The listing builds one solid part. Answer for the finished solid, in the listing's coordinates (mm). Coordinates: 2 decimals unless noted, no trailing zeros. Order: outer loops, then holes, each group sorted by start corner. A loop starts at its lowest first (then second) coordinate and runs counter-clockwise, first axis right, second up.
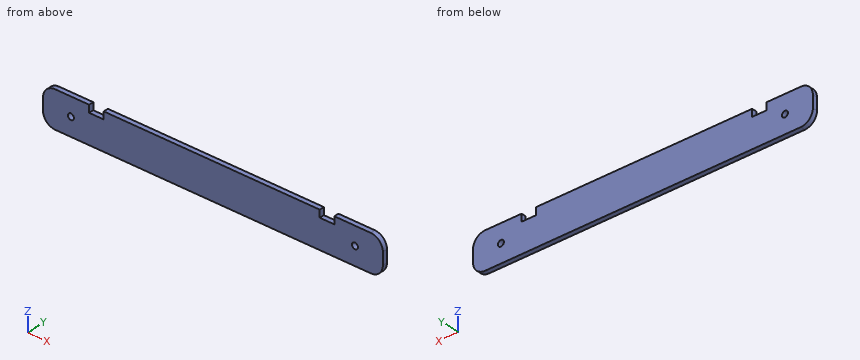
Autodesk Inventor part; units mm, degrees
ref_plane "YZ Plane" through (0, 0, 0) normal (1, 0, 0) x (0, 1, 0)
ref_plane "XZ Plane" through (0, 0, 0) normal (0, 1, 0) x (-1, 0, 0)
ref_plane "XY Plane" through (0, 0, 0) normal (0, 0, 1) x (1, 0, 0)
sketch "Sketch1" plane through (0, 0, 0) normal (0, 1, 0) x (-1, 0, 0)
  line L0 (70, 7.5) -> (-70, 7.5)
  line L1 (-70, 7.5) -> (-70, -7.5)
  line L2 (-70, -7.5) -> (70, -7.5)
  line L3 (70, -7.5) -> (70, 7.5)
  line L4 (51, 7.5) -> (51, 4.5)
  line L5 (51, 4.5) -> (45, 4.5)
  line L6 (45, 4.5) -> (45, 7.5)
  line L7 (-50, 7.5) -> (-50, 4.5)
  line L8 (-50, 4.5) -> (-44, 4.5)
  line L9 (-44, 4.5) -> (-44, 7.5)
  point P0 (0, 0)
  point P1 (58.5, 0)
  point P2 (-58.5, 0)
  point P3 (-70, 0)
  dimension "d0" = 117
  dimension "d1" = 58.5
  dimension "d2" = 140
  dimension "d3" = 70
  dimension "d4" = 7.5
  dimension "d5" = 15
  dimension "d6" = 7.5
  dimension "d7" = 6
  dimension "d8" = 3
  dimension "d9" = 7.5
  dimension "d10" = 6
  dimension "d11" = 3
  dimension "d12" = 101
extrude "Extrusion1" add sketch "Sketch1" along normal blind 2 contours L3 L2 L1 L0 L7 L8 L9 L6 L5 L4
hole "Hole1" at (-58.5, 0, 0) at (58.5, 0, 0) direction (0, 1, 0) diameter 2.5 depth 6.5
fillet "Fillet1" radius 5 4 edges at (-70, 1, 7.5) (-70, 1, -7.5) (70, 1, 7.5) (70, 1, -7.5)
properties part number "3DP_PLA_Screw_Spacing_Test_Part"
(1) Find the intervals of material crossed by probe 1 along X at (y, z) = (0.8, 0); probe 2 along X at (y, z) = (0.55, -1); probe 3 along Z at (x, y) = (58.5, 0.7), in increasing order.
(2) Find section D-D on x = -47.5. Determine the outline of the cut face in (y, z), then the cut area to 3 significant figures.
(3) Find section C-C on y = 1.3. Determine the outline of the cut face in (x, z).
(4) Find section B-B on z = 0. Determine the outline of the cut face in (x, y), then the cut area to 3 significant figures.
(5) Given pin 1 Ø0.6 at (y, z) = (1, 6) entering from -X; pin 2 Ø2 at (x, z) = (-58.5, 0) entering from -Y; pin 3 Ø3 at (x, z) = (58.5, 0) entering from -Y; pin 4 Ø0.6 at (x, y) = (46.5, 1) entering from +Z, each flat-ended and moving along its own axis, determine where each tip first touches the part or whether it passes through.
(6) Find section A-A on x = 58.5. Determine the outline of the cut face in (y, z).
Resolved:
1. probe 1: x = -70 to -59.75, -57.25 to 57.25, 59.75 to 70
1. probe 2: x = -70 to -59.25, -57.75 to 57.75, 59.25 to 70
1. probe 3: z = -7.5 to -1.25, 1.25 to 7.5
2. outline: (0, -7.5) - (2, -7.5) - (2, 4.5) - (0, 4.5) - close
2. area: 24.0 mm2
3. outline: (-70, -2.5) arc R5 ccw to (-65, -7.5) - (65, -7.5) arc R5 ccw to (70, -2.5) - (70, 2.5) arc R5 ccw to (65, 7.5) - (50, 7.5) - (50, 4.5) - (44, 4.5) - (44, 7.5) - (-45, 7.5) - (-45, 4.5) - (-51, 4.5) - (-51, 7.5) - (-65, 7.5) arc R5 ccw to (-70, 2.5) - close; hole circle Ø2.5 at (-58.5, 0); hole circle Ø2.5 at (58.5, 0)
4. outline: (-70, 0) - (-59.75, 0) - (-59.75, 2) - (-70, 2) - close; (-57.25, 0) - (57.25, 0) - (57.25, 2) - (-57.25, 2) - close; (59.75, 0) - (70, 0) - (70, 2) - (59.75, 2) - close
4. area: 270 mm2
5. pin 1: stops at x = -68.84
5. pin 2: passes through
5. pin 3: stops at y = 0
5. pin 4: stops at z = 4.5
6. outline: (0, -7.5) - (2, -7.5) - (2, -1.25) - (0, -1.25) - close; (0, 1.25) - (2, 1.25) - (2, 7.5) - (0, 7.5) - close
